```python
from build123d import *

# Parameters (mm, degrees)
BOSS_EXTRUDE2_DEPTH     = 25
BOSS_EXTRUDE2_2_DEPTH   = 25
SKETCH1_4_W             = 176
SKETCH1_4_H             = 90
BOSS_EXTRUDE3_DEPTH     = 19
BOSS_EXTRUDE4_DEPTH     = 12
FILLET2_R               = 5
CUT_EXTRUDE3_DEPTH      = 6
CUT_EXTRUDE4_DEPTH      = 222.076909694
CUT_EXTRUDE4_DEPTH_BACK = 222.076909694
SKETCH7_W               = 7
SKETCH7_H               = 6
M8_TAPPED_HOLE1_D       = 6.8


with BuildPart() as part:
    # Sketch1 → Boss-Extrude2 (new body)
    with BuildSketch(Plane(origin=(0, 0, 0), x_dir=(1, 0, 0), z_dir=(0, 1, 0))):
        Polygon((-95, 45), (-95, 25), (-95, -25), (-95, -45), (-88, -45), (-88, 45), align=None)
    extrude(amount=BOSS_EXTRUDE2_DEPTH)



with BuildPart() as body_2:
    # Sketch1 → Boss-Extrude2 2 (new body)
    with BuildSketch(Plane(origin=(0, 0, 0), x_dir=(1, 0, 0), z_dir=(0, 1, 0))):
        Polygon((95, 45), (88, 45), (88, -45), (95, -45), (95, -25), (95, 25), align=None)
    extrude(amount=BOSS_EXTRUDE2_2_DEPTH)


with BuildPart() as part_1:
    add(part.part)

    add(body_2.part)  # Boss-Extrude3 merges body 2
    # Sketch1<4> → Boss-Extrude3 (add)
    # profile 1 of 2: a face of its own
    with BuildSketch(Plane(origin=(0, 0, 0), x_dir=(1, 0, 0), z_dir=(0, 1, 0))):
        Rectangle(SKETCH1_4_W, SKETCH1_4_H)
        with BuildLine():
            Line((77, -30), (-77, -30))
            ThreePointArc((-77, -30), (-80.535533906, -28.535533906), (-82, -25))
            Line((-82, -25), (-82, 25))
            ThreePointArc((-82, 25), (-80.535533906, 28.535533906), (-77, 30))
            Line((-77, 30), (77, 30))
            ThreePointArc((77, 30), (80.535533906, 28.535533906), (82, 25))
            Line((82, 25), (82, -25))
            ThreePointArc((82, -25), (80.535533906, -28.535533906), (77, -30))
        make_face(mode=Mode.SUBTRACT)
    # profile 2 of 2: a face of its own
    with BuildSketch(Plane(origin=(0, 0, 0), x_dir=(1, 0, 0), z_dir=(0, 1, 0))):
        with BuildLine():
            ThreePointArc((-82, 25), (-80.535533906, 28.535533906), (-77, 30))
            Line((-77, 30), (77, 30))
            ThreePointArc((77, 30), (80.535533906, 28.535533906), (82, 25))
            Line((82, 25), (82, -25))
            ThreePointArc((82, -25), (80.535533906, -28.535533906), (77, -30))
            Line((77, -30), (-77, -30))
            ThreePointArc((-77, -30), (-80.535533906, -28.535533906), (-82, -25))
            Line((-82, -25), (-82, 25))
        make_face()
    extrude(amount=BOSS_EXTRUDE3_DEPTH)

    # Sketch1<5> → Boss-Extrude4 (add)
    with BuildSketch(Plane(origin=(0, 0, 0), x_dir=(1, 0, 0), z_dir=(0, 1, 0))):
        with BuildLine():
            Line((115, 25), (95, 25))
            Line((95, 25), (95, -25))
            Line((95, -25), (115, -25))
            ThreePointArc((115, -25), (118.535533906, -23.535533906), (120, -20))
            Line((120, -20), (120, -7))
            Line((120, -7), (108, -7))
            ThreePointArc((108, -7), (101, 0), (108, 7))
            Line((108, 7), (120, 7))
            Line((120, 7), (120, 20))
            ThreePointArc((120, 20), (118.535533906, 23.535533906), (115, 25))
        make_face()
        with BuildLine():
            Line((-95, -25), (-95, 25))
            Line((-95, 25), (-115, 25))
            ThreePointArc((-115, 25), (-118.535533906, 23.535533906), (-120, 20))
            Line((-120, 20), (-120, 7))
            Line((-120, 7), (-108, 7))
            ThreePointArc((-108, 7), (-101, 0), (-108, -7))
            Line((-108, -7), (-120, -7))
            Line((-120, -7), (-120, -20))
            ThreePointArc((-120, -20), (-118.535533906, -23.535533906), (-115, -25))
            Line((-115, -25), (-95, -25))
        make_face()
    extrude(amount=BOSS_EXTRUDE4_DEPTH)

    # Fillet2
    fillet2_edges = [part_1.edges().sort_by_distance(p)[0] for p in [
        (95, 6, -25),
        (95, 6, 25),
        (-95, 6, 25),
        (-95, 6, -25),
    ]]
    fillet(fillet2_edges, radius=FILLET2_R)

    # Sketch1<6> → Cut-Extrude3 (cut)
    with BuildSketch(Plane(origin=(0, 0, 0), x_dir=(1, 0, 0), z_dir=(0, 1, 0))):
        with BuildLine():
            ThreePointArc((-82, 25), (-80.535533906, 28.535533906), (-77, 30))
            Line((-77, 30), (77, 30))
            ThreePointArc((77, 30), (80.535533906, 28.535533906), (82, 25))
            Line((82, 25), (82, -25))
            ThreePointArc((82, -25), (80.535533906, -28.535533906), (77, -30))
            Line((77, -30), (-77, -30))
            ThreePointArc((-77, -30), (-80.535533906, -28.535533906), (-82, -25))
            Line((-82, -25), (-82, 25))
        make_face()
    extrude(amount=CUT_EXTRUDE3_DEPTH, mode=Mode.SUBTRACT)

    # Sketch7 → Cut-Extrude4 (cut, two sides: drawn at the far end of the back side and taken through both)
    with BuildSketch(Plane.ZY.offset(95).offset(-CUT_EXTRUDE4_DEPTH_BACK)):
        with Locations((41.5, 9)):
            Rectangle(SKETCH7_W, SKETCH7_H)
        with Locations((-41.5, 9)):
            Rectangle(SKETCH7_W, SKETCH7_H)
    extrude(amount=CUT_EXTRUDE4_DEPTH + CUT_EXTRUDE4_DEPTH_BACK, mode=Mode.SUBTRACT)

    # M8 Tapped Hole1 (through all)
    with Locations(Plane(origin=(0, 19, 0), x_dir=(1, 0, 0), z_dir=(0, 1, 0))):
        with Locations((-72, 25), (72, 25), (72, -25), (-72, -25)):
            Hole(M8_TAPPED_HOLE1_D / 2)


solid = part_1.part
```
Check sheet for the modelled part. Datum: model origin and axes. Units: mm. A direction names the side the tool comes from. Round coordinates to 2 decimals unless told otherwise and drop trailing zeros. Order: outer loops, then holes, each group sorted by start corner. A loop starts at its lowest first (then second) coordinate and runs counter-clockwise, first axis right, second up. Notation, with made-up numbers: M -12.5,40 L -7.5,40 A6 cw -7.5,49 Z; hole C -20.75,89.25 d1. An arc over 180 degrees is marked long. Answer in a Markdown table with one row per item.
(1) Set-up check for faces 1 (the flat face through (82, 3, 0)), 2 (the flat face through (-1, 19, -1)), 3 (the flat face through (-114, 6, -7)), 4 (the flat face through (1, 12, 41)), 5 (the flat face through (1, 6, -42)): record each of +Z, -Z, +X, -X, +Y, -Y from which the full face is reachable in a straight line by a thin tool's end or side.
Findings:
| item | result |
|---|---|
| face 1 | -Y |
| face 2 | +Z, -Z, +Y |
| face 3 | -X, +Y, -Y |
| face 4 | +Z, +X, -X |
| face 5 | -Z, +X, -X |
(2) Draft check along X on faces 6 (the cylindrical face through (74.506, 12.409, 22.702)), 7 (the flat face through (-114, 6, 7)), 8 (the flat face through (120, 6, 14)). Enter one of: +X half, -X half, draft (parallel to the pull), parting line (faces both ways), or undercut.
Findings:
| item | result |
|---|---|
| face 6 | undercut |
| face 7 | draft |
| face 8 | +X half |
(3) Section check D-D on x = 28.5. Record the boundary of the cut face in (y, z).
Findings:
| item | result |
|---|---|
| outline | M 0,-45 L 6,-45 L 6,-38 L 12,-38 L 12,-45 L 19,-45 L 19,45 L 12,45 L 12,38 L 6,38 L 6,45 L 0,45 L 0,30 L 6,30 L 6,-30 L 0,-30 Z |
(4) Gauge pin test, flat ends, axial feed: pin 1 (5.5 mm diameter, centred on x = -35, z = 41.5, fed in from +Y); pin 2 (9.5 mm diameter, centred on x = -107, y = 3.5, fed in from -Z); pin 3 (1.8 mm diameter, centred on x = 27, y = 7.5, fed in from -Z). Record the tip position at first contact, or that the pin passes through.
Findings:
| item | result |
|---|---|
| pin 1 | stops at y = 19 |
| pin 2 | stops at z = -25 |
| pin 3 | stops at z = -38 |
(5) Section check A-A on y = 22.5. Record the boundary of the cut face in (x, z), plus the area to 3 significant figures.
Findings:
| item | result |
|---|---|
| outline | M -95,-45 L -88,-45 L -88,45 L -95,45 Z; M 88,-45 L 95,-45 L 95,45 L 88,45 Z |
| area | 1,260 mm^2 |
(6) Section check C-C on z = 11. Record the boundary of the cut face in (x, y).
Findings:
| item | result |
|---|---|
| outline | M -120,0 L -82,0 L -82,6 L 82,6 L 82,0 L 120,0 L 120,12 L 95,12 L 95,25 L 88,25 L 88,19 L -88,19 L -88,25 L -95,25 L -95,12 L -120,12 Z |
(7) Section check B-B on x = 72. Record the boundary of the cut face in (y, z).
Findings:
| item | result |
|---|---|
| outline | M 0,-45 L 6,-45 L 6,-38 L 12,-38 L 12,-45 L 19,-45 L 19,-28.4 L 6,-28.4 L 6,-30 L 0,-30 Z; M 0,30 L 6,30 L 6,28.4 L 19,28.4 L 19,45 L 12,45 L 12,38 L 6,38 L 6,45 L 0,45 Z; M 6,-21.6 L 19,-21.6 L 19,21.6 L 6,21.6 Z |
(8) Material ranges on line 1 along X through (y, z) = (13.25, -25); line 2 along Z through (x, y) = (-72, 13.75); line 3 along X through (y, z) = (14.5, 26.5), recorded low to high. Write a range as from..to.
Findings:
| item | result |
|---|---|
| line 1 | x = -95..-75.4, -68.6..68.6, 75.4..95 |
| line 2 | z = -45..-28.4, -21.6..21.6, 28.4..45 |
| line 3 | x = -95..-75.05, -68.95..68.95, 75.05..95 |
